The listing builds one solid part. Answer for the finished solid, in the listing's coordinates (mm). Face numbers are marked on the shaded views. A direction names the side the tool comes from. Give positions to 0.01 mm unless a question says otherwise; leave off trailing zeros. Order: outer loops, then holes, each group sorted by start corner. A loop starts at its lowest first (then second) coordinate and runs counter-clockwise, first axis right, second up.
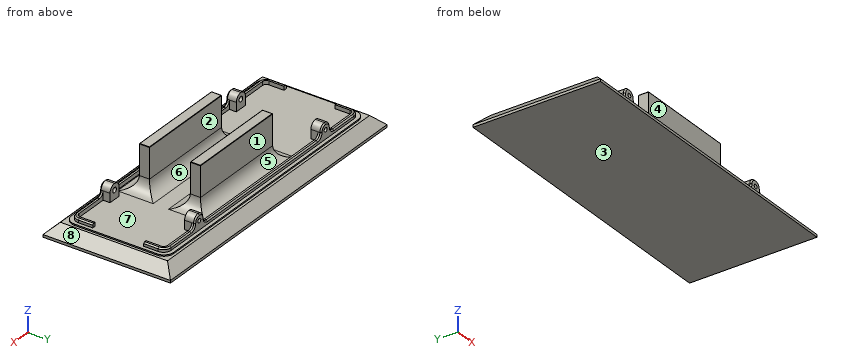
```python
from build123d import *

# Parameters (mm, degrees)
SKETCH_W        = 220
SKETCH_H        = 80
PAD_DEPTH       = 1
SKETCH001_W     = 214.5
SKETCH001_H     = 74.5
SKETCH001_W_2   = 209.5
SKETCH001_H_2   = 69.5
PAD001_DEPTH    = 3
SKETCH002_W     = 2.5
SKETCH002_H     = 40
POCKET_DEPTH    = 3
SKETCH003_W     = 10
SKETCH003_H     = 8
PAD002_DEPTH    = 12
SKETCH008_W     = 80
SKETCH008_H     = 8
PAD003_DEPTH    = 33.8
SKETCH007_W     = 240
SKETCH007_H     = 100
PAD004_DEPTH    = 10
SKETCH009_R     = 1.6
POCKET001_DEPTH = 80
SKETCH010_R     = 2
POCKET002_DEPTH = 6
SKETCH011_R     = 2
POCKET003_DEPTH = 6
FILLET_R        = 3
FILLET001_R     = 6
FILLET002_R     = 7.5
FILLET003_R     = 4.99
FILLET004_R     = 4
CHAMFER_SIZE    = 1
CHAMFER001_SIZE = 1
FILLET005_R     = 10
FILLET006_R     = 0.3
CHAMFER002_SIZE = 8


with BuildPart() as part:
    # Sketch → Pad (new body)
    with BuildSketch(Plane.XY):
        Rectangle(SKETCH_W, SKETCH_H)
    extrude(amount=PAD_DEPTH)

    # Sketch001 (on Face6 of Pad) → Pad001 (join)
    with BuildSketch(Plane.XY.offset(1)):
        Rectangle(SKETCH001_W, SKETCH001_H)
        Rectangle(SKETCH001_W_2, SKETCH001_H_2, mode=Mode.SUBTRACT)
    extrude(amount=PAD001_DEPTH)

    # Sketch002 (on Face11 of Pad001) → Pocket (cut)
    with BuildSketch(Plane.XY.offset(4)):
        with Locations((-106, 0)):
            Rectangle(SKETCH002_W, SKETCH002_H)
        with Locations((106, 0)):
            Rectangle(SKETCH002_W, SKETCH002_H)
    extrude(amount=-POCKET_DEPTH, mode=Mode.SUBTRACT)

    # Sketch003 → Pad002 (join)
    with BuildSketch(Plane.XY.offset(1)):
        with Locations((-70, 33.25)):
            Rectangle(SKETCH003_W, SKETCH003_H)
        with Locations((70, 33.25)):
            Rectangle(SKETCH003_W, SKETCH003_H)
        with Locations((70, -33.25)):
            Rectangle(SKETCH003_W, SKETCH003_H)
        with Locations((-70, -33.25)):
            Rectangle(SKETCH003_W, SKETCH003_H)
    extrude(amount=PAD002_DEPTH)

    # Sketch008 → Pad003 (join)
    with BuildSketch(Plane.XY.offset(1)):
        with Locations((10, 20)):
            Rectangle(SKETCH008_W, SKETCH008_H)
        with Locations((10, -20)):
            Rectangle(SKETCH008_W, SKETCH008_H)
    extrude(amount=PAD003_DEPTH)

    # Sketch007 → Pad004 (join)
    with BuildSketch(Plane(origin=(0, 0, 0), x_dir=(1, 0, 0), z_dir=(0, 0, -1))):
        Rectangle(SKETCH007_W, SKETCH007_H)
    extrude(amount=PAD004_DEPTH)

    # Sketch009 (on Face13 of Pad004) → Pocket001 (cut)
    with BuildSketch(Plane.XZ.offset(37.25)):
        with Locations((-70, 8)):
            Circle(SKETCH009_R)
        with Locations((70, 8)):
            Circle(SKETCH009_R)
    extrude(amount=-POCKET001_DEPTH, mode=Mode.SUBTRACT)

    # Sketch010 (on Face25 of Pocket001) → Pocket002 (cut)
    with BuildSketch(Plane(origin=(0, -29.25, 0), x_dir=(-1, 0, 0), z_dir=(0, 1, 0))):
        with Locations((-70, 8)):
            Circle(SKETCH010_R)
        with Locations((70, 8)):
            Circle(SKETCH010_R)
    extrude(amount=-POCKET002_DEPTH, mode=Mode.SUBTRACT)

    # Sketch011 (on Face48 of Pocket002) → Pocket003 (cut)
    with BuildSketch(Plane.XZ.offset(-29.25)):
        with Locations((-70, 8)):
            Circle(SKETCH011_R)
        with Locations((70, 8)):
            Circle(SKETCH011_R)
    extrude(amount=-POCKET003_DEPTH, mode=Mode.SUBTRACT)

    # Fillet
    fillet_edges = [part.edges().sort_by_distance(p)[0] for p in [
        (104.75, -34.75, 2.5),
        (104.75, 34.75, 2.5),
        (-104.75, -34.75, 2.5),
        (-104.75, 34.75, 2.5),
    ]]
    fillet(fillet_edges, radius=FILLET_R)

    # Fillet001
    fillet001_edges = [part.edges().sort_by_distance(p)[0] for p in [
        (-107.25, 37.25, 2.5),
        (-107.25, -37.25, 2.5),
        (107.25, 37.25, 2.5),
        (107.25, -37.25, 2.5),
    ]]
    fillet(fillet001_edges, radius=FILLET001_R)

    # Fillet002
    fillet002_edges = [part.edges().sort_by_distance(p)[0] for p in [
        (110, 40, 0.5),
        (-110, 40, 0.5),
        (110, -40, 0.5),
        (-110, -40, 0.5),
    ]]
    fillet(fillet002_edges, radius=FILLET002_R)

    # Fillet003
    fillet003_edges = [part.edges().sort_by_distance(p)[0] for p in [
        (75, 33.25, 13),
        (65, 33.25, 13),
        (75, -33.25, 13),
        (65, -33.25, 13),
        (-65, 33.25, 13),
        (-75, 33.25, 13),
        (-65, -33.25, 13),
        (-75, -33.25, 13),
    ]]
    fillet(fillet003_edges, radius=FILLET003_R)

    # Fillet004
    fillet004_edges = [part.edges().sort_by_distance(p)[0] for p in [
        (75, 36, 4),
        (75, -36, 4),
        (-65, -36, 4),
        (-65, 36, 4),
        (-75, 36, 4),
        (-75, -36, 4),
        (65, -36, 4),
        (65, 36, 4),
    ]]
    fillet(fillet004_edges, radius=FILLET004_R)

    # Chamfer
    chamfer_edges = [part.edges().sort_by_distance(p)[0] for p in [
        (66.461537, -37.25, 11.538463),
    ]]
    chamfer(chamfer_edges, length=CHAMFER_SIZE)

    # Chamfer001
    chamfer001_edges = [part.edges().sort_by_distance(p)[0] for p in [
        (-73.538463, 37.25, 11.538463),
    ]]
    chamfer(chamfer001_edges, length=CHAMFER001_SIZE)

    # Fillet005
    fillet005_edges = [part.edges().sort_by_distance(p)[0] for p in [
        (10, 24, 1),
        (50, 20, 1),
        (50, -20, 1),
        (10, -16, 1),
        (-30, 20, 1),
        (10, 16, 1),
        (-30, -20, 1),
        (10, -24, 1),
    ]]
    fillet(fillet005_edges, radius=FILLET005_R)

    # Fillet006
    fillet006_edges = [part.edges().sort_by_distance(p)[0] for p in [
        (-30, -20, 34.8),
        (-30, 20, 34.8),
        (50, 20, 34.8),
        (50, -20, 34.8),
        (10, -16, 34.8),
        (10, -24, 34.8),
        (10, 16, 34.8),
        (10, 24, 34.8),
    ]]
    fillet(fillet006_edges, radius=FILLET006_R)

    # Chamfer002
    chamfer002_edges = [part.edges().sort_by_distance(p)[0] for p in [
        (0, -50, 0),
        (-120, 0, 0),
        (0, 50, 0),
        (120, 0, 0),
    ]]
    chamfer(chamfer002_edges, length=CHAMFER002_SIZE)


solid = part.part
```
1) For a pull along X with two mould halves and no side action, classify the marked faces 6, 7 and 8 as +X half, -X half, draft (parallel to the pull), parting line (faces both ways), or undercut.
Geometry says:
face 6: draft
face 7: undercut
face 8: +X half
2) Find section C-C (z = -3). Write down the section's boundary in (x, y).
Geometry says:
outline: (-115, -45) - (115, -45) - (115, 45) - (-115, 45) - close
3) Find section B-B (y = 2). Write down the section's boundary in (x, z).
Geometry says:
outline: (-120, -10) - (120, -10) - (120, -8) - (112, 0) - (110, 0) - (110, 1) - (-110, 1) - (-110, 0) - (-112, 0) - (-120, -8) - close
4) A tool of negligible diameter and unlimited length cuts with its end or side. For the marked faces 1, 2, 3, 4 and 5, from which of +Z, -Z, +X, -X, +Y, -Y can it reach the whole face along a straight path? Write none if from no direction.
Geometry says:
face 1: +Z, +X, -X, +Y
face 2: +Z, +X, -X
face 3: -Z, +X, -X, +Y, -Y
face 4: +Z, +X, -X, -Y
face 5: +Z
5) Straight lines are drawn through the part: probe 1 along Y at (x, z) = (34.5, 26.5); probe 2 along X at (y, z) = (22, 3.5); probe 3 along Z at (x, y) = (-70, 36). For each, find the intervals that lie inside material, in ascending order.
Geometry says:
probe 1: y = -24 to -16, 16 to 24
probe 2: x = -106.75 to -104.75, -33.39 to 53.39, 104.75 to 106.75
probe 3: z = -10 to 6.4, 9.6 to 13
6) Find section A-A (z = 24.5). Write down the section's boundary in (x, y), then the cut area to 3 significant figures.
Geometry says:
outline: (-30, -24) - (50, -24) - (50, -16) - (-30, -16) - close; (-30, 16) - (50, 16) - (50, 24) - (-30, 24) - close
area: 1,280 mm2
7) Find section D-D (y = -10). Write down the section's boundary in (x, z).
Geometry says:
outline: (-120, -10) - (120, -10) - (120, -8) - (112, 0) - (110, 0) - (110, 1) - (60, 1) arc R10 cw to (56, 1.83) - (-36, 1.83) arc R10 cw to (-40, 1) - (-110, 1) - (-110, 0) - (-112, 0) - (-120, -8) - close
8) Given P1, Ø2, axis at y = 31, z = 5.5, coming from the +X side; P2, Ø6.5, axis at x = 70, z = 8, coming from the -Y side; P3, Ø5, axis at x = 72, z = 6.5, coming from the +Y side, each flat-ended and moving along its own axis, determine where each tip first touches the part or whether it passes through.
Geometry says:
P1: stops at x = 75
P2: stops at y = -37.25
P3: stops at y = 37.25
